Verification items for the finished model (mm, model axes). A direction names the side the tool comes from. Give positions to 0.01 mm unless a question says otherwise; leave off trailing zeros. Order: outer loops, then holes, each group sorted by start corner. A loop starts at its lowest first (then second) coordinate and runs counter-clockwise, first axis right, second up.
from build123d import *

# Parameters (mm, degrees)
SKETCH_1_W      = 39
SKETCH_1_H      = 69
EXTRUDE_1_DEPTH = 1.5
SKETCH_2_R      = 3.5
SKETCH_2_R_2    = 1.5
EXTRUDE_2_DEPTH = 7


with BuildPart() as part:
    # Эскиз1 → Бобышка-Вытянуть1 (new body)
    with BuildSketch(Plane.XY):
        with Locations((19.5, 34.5)):
            Rectangle(SKETCH_1_W, SKETCH_1_H)
    extrude(amount=EXTRUDE_1_DEPTH)

    # Эскиз2 → Бобышка-Вытянуть2 (add)
    # profile 1 of 3: a face of its own
    with BuildSketch(Plane(origin=(0, 0, 0), x_dir=(-1, 0, 0), z_dir=(0, 0, -1))):
        with Locations((-19, 65.2)):
            Circle(SKETCH_2_R)
        with Locations((-19, 65.2)):
            Circle(SKETCH_2_R_2, mode=Mode.SUBTRACT)
    # profile 2 of 3: a face of its own
    with BuildSketch(Plane(origin=(0, 0, 0), x_dir=(-1, 0, 0), z_dir=(0, 0, -1))):
        with Locations((-35, 23)):
            Circle(SKETCH_2_R)
        with Locations((-35, 23)):
            Circle(SKETCH_2_R_2, mode=Mode.SUBTRACT)
    # profile 3 of 3: a face of its own
    with BuildSketch(Plane(origin=(0, 0, 0), x_dir=(-1, 0, 0), z_dir=(0, 0, -1))):
        with Locations((-19, 12.2)):
            Circle(SKETCH_2_R)
        with Locations((-19, 12.2)):
            Circle(SKETCH_2_R_2, mode=Mode.SUBTRACT)
    extrude(amount=EXTRUDE_2_DEPTH)


solid = part.part
(1) Go/stop test with flat-tipped pins: pin 1 (0.9 mm diameter, centred on x = 19, y = 12.5, fed in from -Z); pin 2 (1 mm diameter, centred on x = 13, z = -2, fed in from +Y); pin 3 (2 mm diameter, centred on y = 26, z = -3, fed in from +X). Record where each tip stops, or that it passes through.
Solved:
pin 1: stops at z = 0
pin 2: passes through
pin 3: stops at x = 37.87
(2) Set-up check for faces 5 (the flat face through (35, 21, -7)), 6 (the cylindrical face through (17.385, 62.095, -3.451)): record each of +Z, -Z, +X, -X, +Y, -Y from which the full face is reachable in a straight line by a thin tool's end or side.
Solved:
face 5: -Z, +X, -X, +Y, -Y
face 6: -Z
(3) Scan lines: line 1 (Y direction, x = 19, z = -3); line 2 (Y direction, x = 35, z = -5.5); line 3 (Z direction, x = 5, y = 39). Record each from-to range of solid material in increasing order.
Solved:
line 1: y = 8.7 to 10.7, 13.7 to 15.7, 61.7 to 63.7, 66.7 to 68.7
line 2: y = 19.5 to 21.5, 24.5 to 26.5
line 3: z = 0 to 1.5
(4) Release check for a two-part mould opening along X. For faces 1 (the cylindrical face through (20.5, 12.27, -3.45)), 2 (the cylindrical face through (37.58, 25.365, -3.451)), 3 (the flat face through (35, 23, 0)), 4 (the flat face through (0, 34, 1)) record: pulls with the +X half, pulls with the -X half, needs draft (parallel to the pull), parting line crosses it, or undercut.
Solved:
face 1: undercut
face 2: parting line crosses it
face 3: undercut
face 4: pulls with the -X half
(5) Section check D-D, the plane x = 19. Enter the section's corners in (y, z), then the cut area to 4 significant figures.
Solved:
outline: (0, 0) - (8.7, 0) - (8.7, -7) - (10.7, -7) - (10.7, 0) - (13.7, 0) - (13.7, -7) - (15.7, -7) - (15.7, 0) - (61.7, 0) - (61.7, -7) - (63.7, -7) - (63.7, 0) - (66.7, 0) - (66.7, -7) - (68.7, -7) - (68.7, 0) - (69, 0) - (69, 1.5) - (0, 1.5) - close
area: 159.5 mm2
(6) Section check A-A, the plane z = -2.25. Enter the section's corners in (x, y).
Solved:
outline: circle Ø7 at (19, 12.2); circle Ø7 at (19, 65.2); circle Ø7 at (35, 23); hole circle Ø3 at (19, 12.2); hole circle Ø3 at (19, 65.2); hole circle Ø3 at (35, 23)
(7) Section check B-B, the plane y = 12.2. Enter the section's corners in (x, z).
Solved:
outline: (0, 0) - (15.5, 0) - (15.5, -7) - (17.5, -7) - (17.5, 0) - (20.5, 0) - (20.5, -7) - (22.5, -7) - (22.5, 0) - (39, 0) - (39, 1.5) - (0, 1.5) - close
(8) Section check C-C, the plane x = 35. Enter the section's corners in (y, z), then the cut area to 4 significant figures.
Solved:
outline: (0, 0) - (19.5, 0) - (19.5, -7) - (21.5, -7) - (21.5, 0) - (24.5, 0) - (24.5, -7) - (26.5, -7) - (26.5, 0) - (69, 0) - (69, 1.5) - (0, 1.5) - close
area: 131.5 mm2
